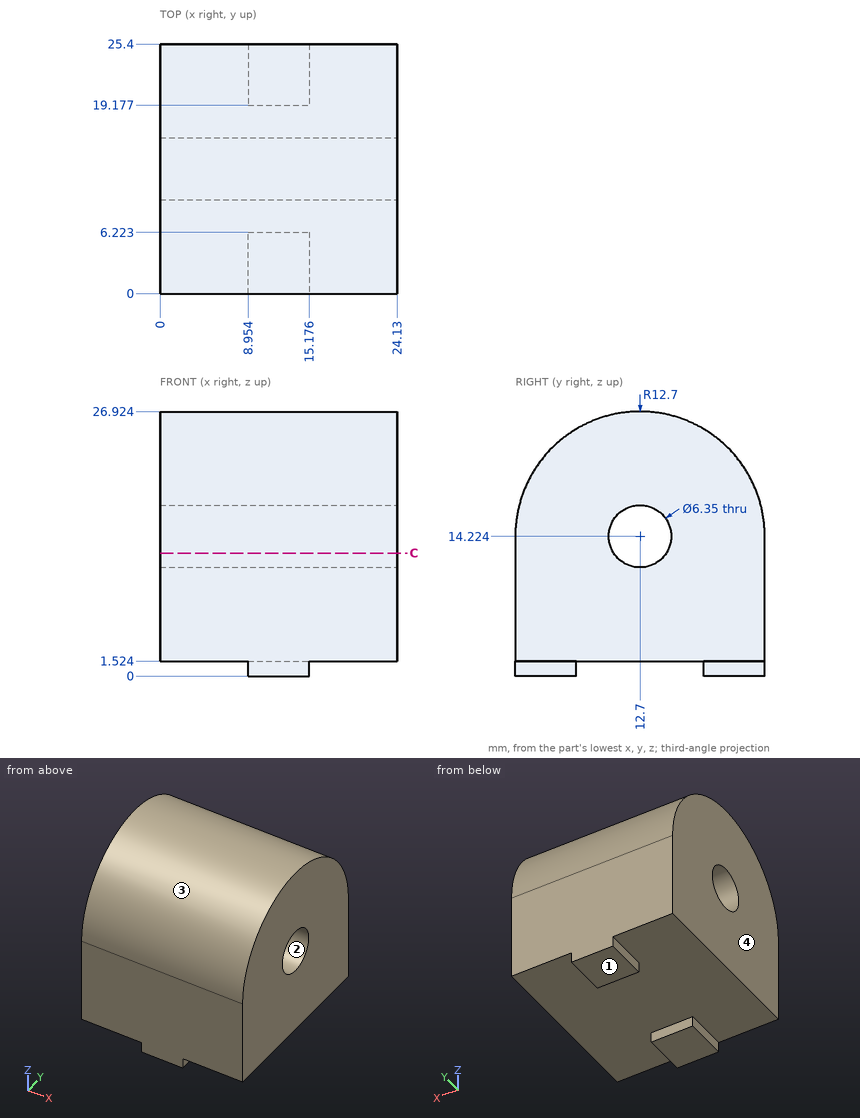
Input: dimensioned drawing with shaded views. Units: mm. Origin: part minimum x, y, z. Round coordinates to 2 decimals unless told otherwise and drop trailing zeros. Loops run counter-clockwise (first coordinate to the right, second up) from the corner with the lowest first, then second, coordinate; pieces in that order, holes last. Notation, with made-up numbers: (38.5, 41) -> (60.5, 41) arc R31 cw to (60.5, 74) -> close; hole circle Ø6 at (4, 3.5). An arc over 180 degrees is marked (long way). Answer as a JSON object with one key per item and string values. Group by question number.
1) Section query C-C on z = 12.5. Output: boundary loops of the cut face in (x, y).
2) Draft query along Z for the marked faces 1, 2, 3 and 4. Return one class per face: +Z half, -Z half, draft (parallel to the pull), parting line (faces both ways), or undercut.
3) Ray query, L1, parallel to Z at x = 14, y = 14.25 (1 decimal); L2, parallel to Y at x = 2, z = 14.75; L3, parallel to Y at x = 8.5, z = 15.25 (1 decimal). Return the intervals inside material, ascending.
4) Pin query (flat end, axial travel): pin 1 (6 mm diameter, centred on x = 20, y = 6, fed in from +Z); pin 2 (0.8 mm diameter, centred on y = 23.5, z = 1, fed in from -X); pin 3 (1 mm diameter, centred on x = 11.5, y = 17.5, fed in from +Z). Return the tip coordinate at first contact, or that it passes through.
Reply:
{
 "1": {"outline": "(0, 0) -> (24.13, 0) -> (24.13, 10.03) -> (0, 10.03) -> close; (0, 15.37) -> (24.13, 15.37) -> (24.13, 25.4) -> (0, 25.4) -> close"},
 "2": {"face 1": "-Z half", "face 2": "undercut", "face 3": "+Z half", "face 4": "draft"},
 "3": {"L1": "z = 1.5 to 11.5, 17 to 26.8", "L2": "y = 0.01 to 9.57, 15.83 to 25.39", "L3": "y = 0 to 9.7, 15.7 to 25.4"},
 "4": {"pin 1": "stops at z = 26.37", "pin 2": "stops at x = 8.95", "pin 3": "stops at z = 26.17"}
}
